Autodesk Inventor part; units mm, degrees
ref_plane "YZ Plane" through (0, 0, 0) normal (1, 0, 0) x (0, 1, 0)
ref_plane "XZ Plane" through (0, 0, 0) normal (0, 1, 0) x (-1, 0, 0)
ref_plane "XY Plane" through (0, 0, 0) normal (0, 0, 1) x (1, 0, 0)
sketch "スケッチ1" plane through (0, 0, 0) normal (0, 1, 0) x (-1, 0, 0)
  line L0 (-88.25, 46.25) -> (88.25, 46.25)
  line L1 (88.25, 46.25) -> (88.25, -46.25)
  line L2 (88.25, -46.25) -> (-88.25, -46.25)
  line L3 (-88.25, -46.25) -> (-88.25, 46.25)
  line L4 (-88.25, 46.25) -> (88.25, -46.25) construction
  line L5 (88.25, 46.25) -> (-88.25, -46.25) construction
  circle A0 centre (84.75, 42.75) radius 1.55
  circle A1 centre (9.75, 42.75) radius 1.55
  circle A2 centre (-84.75, 42.75) radius 1.55
  line L6 (151.0272, 0) -> (-157.6431, 0) construction
  line L7 (0, 129.3763) -> (0, -94.6315) construction
  circle A3 centre (84.75, -42.75) radius 1.55
  circle A4 centre (9.75, -42.75) radius 1.55
  circle A5 centre (-84.75, -42.75) radius 1.55
  circle A6 centre (27.5, -25.75) radius 1.55
  circle A7 centre (27.5, -16.25) radius 1.55
  line L8 (88.25, -25.75) -> (-88.25, -25.75) construction
  line L9 (-88.25, -16.25) -> (88.25, -16.25) construction
  circle A8 centre (-69.5, -25.75) radius 1.55
  circle A9 centre (-69.5, -16.25) radius 1.55
  circle A10 centre (84.75, -29.75) radius 1.55
  circle A11 centre (84.75, -14.75) radius 1.55
  circle A12 centre (84.75, 0.25) radius 1.55
  circle A13 centre (84.75, 15.25) radius 1.55
  circle A14 centre (84.75, 30.25) radius 1.55
  circle A15 centre (76.5, -25.75) radius 1.55
  circle A16 centre (76.5, -13.75) radius 1.55
  circle A17 centre (76.5, -1.75) radius 1.55
  circle A18 centre (76.5, 10.25) radius 1.55
  line L10 (-55.5, -30.75) -> (22, -30.75)
  line L11 (22, -30.75) -> (22, 29.25)
  line L12 (22, 29.25) -> (-55.5, 29.25)
  line L13 (-55.5, 29.25) -> (-55.5, -30.75)
  line L14 (-55.5, -30.75) -> (22, 29.25) construction
  line L15 (22, -30.75) -> (-55.5, 29.25) construction
  point P0 (0, 0)
  point P1 (-16.75, -0.75)
  dimension "d105" = 176.5
  dimension "d106" = 92.5
  dimension "d107" = 3.5
  dimension "d108" = 3.5
  dimension "d109" = 3.1
  dimension "d110" = 78.5
  dimension "d111" = 3.5
  dimension "d112" = 3.1
  dimension "d113" = 173
  dimension "d114" = 3.5
  dimension "d115" = 3.1
  dimension "d116" = 46.25
  dimension "d117" = 88.25
  dimension "d118" = 60.75
  dimension "d119" = 20.5
  dimension "d120" = 30
  dimension "d121" = 3.1
  dimension "d122" = 3.1
  dimension "d123" = 60.75
  dimension "d129" = 3.1
  dimension "d130" = 3.1
  dimension "d132" = 9.5
  dimension "d133" = 20.5
  dimension "d134" = 30
  dimension "d136" = 16.5
  dimension "d137" = 3.5
  dimension "d138" = 3.1
  dimension "d141" = 15
  dimension "d146" = 20.5
  dimension "d147" = 11.75
  dimension "d148" = 3.1
  dimension "d151" = 12
  dimension "d156" = 15.5
  dimension "d157" = 75.5
  dimension "d158" = 66.25
  dimension "d159" = 143.75
  dimension "d164" = 97
  dimension "d165" = 157.75
extrude "押し出し1" add sketch "スケッチ1" along normal blind 3
fillet "フィレット1" radius 2 4 edges at (-22, 1.5, 29.25) (-22, 1.5, -30.75) (55.5, 1.5, 29.25) (55.5, 1.5, -30.75)
fillet "フィレット2" radius 3 4 edges at (-88.25, 1.5, 46.25) (-88.25, 1.5, -46.25) (88.25, 1.5, 46.25) (88.25, 1.5, -46.25)
equation "\"d108\" = d107"
equation "\"d111\" = d107"
equation "\"d112\" = d109"
equation "\"d114\" = d111"
equation "\"d115\" = d112"
equation "\"d121\" = d109"
equation "\"d122\" = d109"
equation "\"d123\" = d118"
equation "\"d129\" = d131"
equation "\"d130\" = d131"
equation "\"d138\" = d109"
equation "\"d148\" = d138"
properties part number "Sole_frame" material "GFRC"
Can you work these out from the model? Positions are in its coordinate system, mm. A direction names the side the tool comes from. Coordinates: 2 decimals unless noted, no trailing zeros. Write each loop counter-clockwise with the first axis right and the second up, starting at its lowest first coordinate (ties: lowest second). Pieces come first, ordered by that corner, then holes. Notation, with made-up numbers: (9.5, 61) -> (46.5, 61) arc R30 cw to (46.5, 84) -> close; hole circle Ø6 at (13, -6). An arc over 180 degrees is marked (long way). Write item = value, one per line.
(1) Imagine slicing it at B-B (x = 38). Please give me the cut outline in (y, z).
Verdict:
outline = (0, -46.25) -> (3, -46.25) -> (3, -30.75) -> (0, -30.75) -> close; (0, 29.25) -> (3, 29.25) -> (3, 46.25) -> (0, 46.25) -> close
(2) If I drill on probe 1 along Z at (x, y) = (-9.75, 1.05); probe 2 along Z at (x, y) = (9.5, 0.95); probe 3 along Z at (x, y) = (-76.5, 1), over which ranges is the centre line in solid material (lowest first)?
Verdict:
probe_1 = -46.25 to -44.3, -41.2 to -30.75, 29.25 to 41.2, 44.3 to 46.25
probe_2 = -46.25 to -30.75, 29.25 to 46.25
probe_3 = -46.25 to -27.3, -24.2 to -15.3, -12.2 to -3.3, -0.2 to 8.7, 11.8 to 46.25
(3) For pin 1 (5 mm diameter, centred on x = -76.5, z = 10.25, fed in from -Y); pin 2 (2.5 mm diameter, centred on x = -76.5, z = -13.75, fed in from +Y) (1 decimal), each with a flat end and sliding along its axis, tell me the tip position at first contact or that it passes through.
Verdict:
pin_1 = 0
pin_2 = through
(4) Thinking about a two-plate mould opening in Z: for faces 3 (the face through (87.35, 1.52, 45.39)), 4 (the face through (-9.414, 1.479, 44.263)), 5 (the face through (-1, 1, -46.25)), which applies, +Z half, -Z half, draft (parallel to the pull), parting line (faces both ways), or undercut?
Verdict:
face_3 = +Z half
face_4 = undercut
face_5 = -Z half
(5) Imagine slicing it at A-A (z = 4). Please give me the cut outline in (x, y), and give its area (3 significant figures).
Verdict:
outline = (-88.25, 0) -> (-22, 0) -> (-22, 3) -> (-88.25, 3) -> close; (55.5, 0) -> (88.25, 0) -> (88.25, 3) -> (55.5, 3) -> close
area = 297 mm^2
(6) On a 3-axis mill with a long thin cutter (end or side, diameter ignored), from which of +Z, -Z, +X, -X, +Y, -Y can I reach the whole of each face in a straight line? I mean faces 1 (the face through (-87.39, 1.52, 45.35)), 2 (the face through (55.5, 1, 0)). Say none if no direction works.
Verdict:
face_1 = +Z, -X, +Y, -Y
face_2 = +Y, -Y
(7) Imagine slicing it at C-C (y = 1.15). State how many separate pieces and enclosed holes the cut face has, and give its area (3 significant figures).
Verdict:
separate_pieces = 1
enclosed_holes = 20
area = 11,500 mm^2
